Design review of the part built by this model. Coordinates are the model's own, in mm. A direction names the side the tool comes from. Give positions to 0.01 mm unless a question says otherwise; leave off trailing zeros. Order: outer loops, then holes, each group sorted by start corner. A loop starts at its lowest first (then second) coordinate and runs counter-clockwise, first axis right, second up. Notation, with made-up numbers: (75, -35.75) -> (104, -35.75) arc R18 ccw to (104, -18.75) -> close; hole circle Ø6 at (76.5, 34.5). An arc over 180 degrees is marked (long way). One line per item, written item: value. Start each with the question number.
1) Wall thickness on line 1 along Z through (x, y) = (49, 50.5); line 2 along X through (y, z) = (55.5, 20); line 3 along Z through (x, y) = (65, 57): over which ranges is each line inside the solid? List them lowest first. Write a range as from..to.
2) Tool access review of faces 4 (the face through (28, 66, 20)), 5 (the face through (25, 63, 23)), 6 (the face through (50, 68, 47.5)), 7 (the face through (1.5, 21, 35)): name each direction out of +Z, -Z, +X, -X, +Y, -Y from which nothing blocks a thin tool from reaching the whole face with its end or side.
3) Consider section A-A (x = 47). State the section outline as (y, z) points.
4) For pin 1 (7.5 mm diameter, centred on x = 30.5, z = 64, fed in from -Y); pin 2 (1 mm diameter, centred on y = 12.5, z = 35, fed in from -X); pin 3 (2 mm diameter, centred on x = 40, z = 58.5, fed in from -Y), all flat-tipped, find the tip position at first contact; note any pin that passes through.
5) Consider section B-B (z = 48.5). State the section outline as (x, y) points.
6) Consider section C-C (z = 11). State the section outline as (x, y) points.
7) The part is to be moulded in two halves that separate along Y. For faces 1 (the face through (68, 50.3, 51)), 2 (the face through (34.8, 5.7, 1.5)), 3 (the face through (1, 20, 35)), say which applies: released by +Y, released by -Y, zero draft, split by the parting line, or undercut.
from build123d import *

# Parameters (mm, degrees)
BOX079_W               = 5
BOX079_H               = 29
BOX079_DEPTH           = 34
BOX078_W               = 5
BOX078_H               = 28
BOX078_DEPTH           = 32
BOX077_W               = 8
BOX077_H               = 8.3
BOX077_DEPTH           = 6.3
BOX075_W               = 11
BOX075_H               = 10
BOX075_DEPTH           = 11
BOX066_W               = 3
BOX066_H               = 3.5
BOX066_DEPTH           = 12
BOX065_W               = 3
BOX065_H               = 7.5
BOX065_DEPTH           = 17.78
BOX064_W               = 10
BOX064_H               = 8.5
BOX064_DEPTH           = 7.7
CYLINDER036_R          = 1.75
CYLINDER036_DEPTH      = 15
CYLINDER035_R          = 1.75
CYLINDER035_DEPTH      = 15
BOX035_W               = 8
BOX035_H               = 3
BOX035_DEPTH           = 6
BOX034_W               = 8
BOX034_H               = 3
BOX034_DEPTH           = 6
CYLINDER016_R          = 1.7
CYLINDER016_DEPTH      = 15
CYLINDER016_ROLL_ANGLE = 90
CYLINDER015_R          = 1.7
CYLINDER015_DEPTH      = 15
CYLINDER015_ROLL_ANGLE = 90
BOX031_W               = 39
BOX031_H               = 40
BOX031_DEPTH           = 2
BOX032_W               = 34
BOX032_H               = 40
BOX032_DEPTH           = 7
BOX032_PITCH_ANGLE     = 90
BOX033_W               = 34
BOX033_H               = 40
BOX033_DEPTH           = 4
BOX033_PITCH_ANGLE     = 90
BOX028_W               = 15.5
BOX028_H               = 2
BOX028_DEPTH           = 2.5
BOX027_W               = 15.5
BOX027_H               = 2
BOX027_DEPTH           = 2.5
BOX026_W               = 2
BOX026_H               = 2.5
BOX026_DEPTH           = 14
BOX026_ROLL_ANGLE      = 90
BOX025_W               = 2
BOX025_H               = 2.5
BOX025_DEPTH           = 14
BOX025_ROLL_ANGLE      = 90
BOX024_W               = 2.5
BOX024_H               = 2
BOX024_DEPTH           = 51
BOX024_PITCH_ANGLE     = 90
BOX023_W               = 2.5
BOX023_H               = 2
BOX023_DEPTH           = 51
BOX023_PITCH_ANGLE     = 90
BOX022_W               = 2.5
BOX022_H               = 2
BOX022_DEPTH           = 62
BOX021_W               = 2.5
BOX021_H               = 2
BOX021_DEPTH           = 67
BOX020_W               = 62
BOX020_H               = 62
BOX020_DEPTH           = 62
BOX020_ROLL_ANGLE      = 90
PAD005_DEPTH           = 70
SKETCH010_R            = 8.5
POCKET002004_DEPTH     = 5
SKETCH011_W            = 45
SKETCH011_H            = 32
POCKET002005_DEPTH     = 4
FILLET_R               = 3
CHAMFER007_SIZE        = 1.5


with BuildPart() as cube078:
    # Box079 → Box079 (new body)
    with BuildSketch(Plane(origin=(22, 26, 4.1), x_dir=(1, 0, 0), z_dir=(0, 0, 1))):
        with Locations((2.5, 14.5)):
            Rectangle(BOX079_W, BOX079_H)
    extrude(amount=BOX079_DEPTH)


with BuildPart() as cube077:
    # Box078 → Box078 (new body)
    with BuildSketch(Plane(origin=(59, 26, 4.1), x_dir=(1, 0, 0), z_dir=(0, 0, 1))):
        with Locations((2.5, 14)):
            Rectangle(BOX078_W, BOX078_H)
    extrude(amount=BOX078_DEPTH)


with BuildPart() as cube076:
    # Box077 → Box077 (new body)
    with BuildSketch(Plane(origin=(64, 42, 47.5), x_dir=(1, 0, 0), z_dir=(0, 0, 1))):
        with Locations((4, 4.15)):
            Rectangle(BOX077_W, BOX077_H)
    extrude(amount=BOX077_DEPTH)


with BuildPart() as cube074:
    # Box075 → Box075 (new body)
    with BuildSketch(Plane(origin=(44.5, 62, 47.5), x_dir=(1, 0, 0), z_dir=(0, 0, 1))):
        with Locations((5.5, 5)):
            Rectangle(BOX075_W, BOX075_H)
    extrude(amount=BOX075_DEPTH)


with BuildPart() as cube065:
    # Box066 → Box066 (new body)
    with BuildSketch(Plane(origin=(66, 13.5, 44.5), x_dir=(1, 0, 0), z_dir=(0, 0, 1))):
        with Locations((1.5, 1.75)):
            Rectangle(BOX066_W, BOX066_H)
    extrude(amount=BOX066_DEPTH)


with BuildPart() as cube064:
    # Box065 → Box065 (new body)
    with BuildSketch(Plane(origin=(66, 6, 41.5), x_dir=(1, 0, 0), z_dir=(0, 0, 1))):
        with Locations((1.5, 3.75)):
            Rectangle(BOX065_W, BOX065_H)
    extrude(amount=BOX065_DEPTH)


with BuildPart() as cube063:
    # Box064 → Box064 (new body)
    with BuildSketch(Plane(origin=(60, 4, 46.5), x_dir=(1, 0, 0), z_dir=(0, 0, 1))):
        with Locations((5, 4.25)):
            Rectangle(BOX064_W, BOX064_H)
    extrude(amount=BOX064_DEPTH)


with BuildPart() as cylinder068:
    # Cylinder036 → Cylinder036 (new body)
    with BuildSketch(Plane(origin=(24.5, 13.5, -4), x_dir=(1, 0, 0), z_dir=(0, 0, 1))):
        Circle(CYLINDER036_R)
    extrude(amount=CYLINDER036_DEPTH)


with BuildPart() as cylinder067:
    # Cylinder035 → Cylinder035 (new body)
    with BuildSketch(Plane(origin=(35.5, 13.5, 59), x_dir=(1, 0, 0), z_dir=(0, 0, 1))):
        Circle(CYLINDER035_R)
    extrude(amount=CYLINDER035_DEPTH)


with BuildPart() as cube035:
    # Box035 → Box035 (new body)
    with BuildSketch(Plane(origin=(22, 61, 17), x_dir=(1, 0, 0), z_dir=(0, 0, 1))):
        with Locations((4, 1.5)):
            Rectangle(BOX035_W, BOX035_H)
    extrude(amount=BOX035_DEPTH)


with BuildPart() as cube034:
    # Box034 → Box034 (new body)
    with BuildSketch(Plane(origin=(60, 61, 17), x_dir=(1, 0, 0), z_dir=(0, 0, 1))):
        with Locations((4, 1.5)):
            Rectangle(BOX034_W, BOX034_H)
    extrude(amount=BOX034_DEPTH)


with BuildPart() as cylinder051:
    # Cylinder016 → Cylinder016 (new body)
    with BuildSketch(Plane.XY):
        Circle(CYLINDER016_R)
    extrude(amount=CYLINDER016_DEPTH)


with BuildPart() as cylinder051_1:
    # Cylinder016 roll: moved
    add(cylinder051.part.rotate(Axis((0, 0, 0), (1, 0, 0)), CYLINDER016_ROLL_ANGLE))


with BuildPart() as cylinder051_2:
    # Cylinder016 placement: moved
    add(cylinder051_1.part.moved(Location((26, 67, 20))))


with BuildPart() as cylinder050:
    # Cylinder015 → Cylinder015 (new body)
    with BuildSketch(Plane.XY):
        Circle(CYLINDER015_R)
    extrude(amount=CYLINDER015_DEPTH)


with BuildPart() as cylinder050_1:
    # Cylinder015 roll: moved
    add(cylinder050.part.rotate(Axis((0, 0, 0), (1, 0, 0)), CYLINDER015_ROLL_ANGLE))


with BuildPart() as cylinder050_2:
    # Cylinder015 placement: moved
    add(cylinder050_1.part.moved(Location((65, 67, 20))))


with BuildPart() as cube031:
    # Box031 → Box031 (new body)
    with BuildSketch(Plane(origin=(25, 26, 36), x_dir=(1, 0, 0), z_dir=(0, 0, 1))):
        with Locations((19.5, 20)):
            Rectangle(BOX031_W, BOX031_H)
    extrude(amount=BOX031_DEPTH)


with BuildPart() as cube032:
    # Box032 → Box032 (new body)
    with BuildSketch(Plane.XY):
        with Locations((17, 20)):
            Rectangle(BOX032_W, BOX032_H)
    extrude(amount=BOX032_DEPTH)


with BuildPart() as cube032_1:
    # Box032 pitch: moved
    add(cube032.part.rotate(Axis((0, 0, 0), (0, 1, 0)), BOX032_PITCH_ANGLE))


with BuildPart() as cube032_2:
    # Box032 placement: moved
    add(cube032_1.part.moved(Location((22, 26, 38))))


with BuildPart() as cube033:
    # Box033 → Box033 (new body)
    with BuildSketch(Plane.XY):
        with Locations((17, 20)):
            Rectangle(BOX033_W, BOX033_H)
    extrude(amount=BOX033_DEPTH)


with BuildPart() as cube033_1:
    # Box033 pitch: moved
    add(cube033.part.rotate(Axis((0, 0, 0), (0, 1, 0)), BOX033_PITCH_ANGLE))


with BuildPart() as cube033_2:
    # Box033 placement: moved
    add(cube033_1.part.moved(Location((62, 26, 38))))


with BuildPart() as cube028:
    # Box028 → Box028 (new body)
    with BuildSketch(Plane(origin=(1.5, 20, 66), x_dir=(1, 0, 0), z_dir=(0, 0, 1))):
        with Locations((7.75, 1)):
            Rectangle(BOX028_W, BOX028_H)
    extrude(amount=BOX028_DEPTH)


with BuildPart() as cube027:
    # Box027 → Box027 (new body)
    with BuildSketch(Plane(origin=(1.5, 20, 1.5), x_dir=(1, 0, 0), z_dir=(0, 0, 1))):
        with Locations((7.75, 1)):
            Rectangle(BOX027_W, BOX027_H)
    extrude(amount=BOX027_DEPTH)


with BuildPart() as cube026:
    # Box026 → Box026 (new body)
    with BuildSketch(Plane.XY):
        with Locations((1, 1.25)):
            Rectangle(BOX026_W, BOX026_H)
    extrude(amount=BOX026_DEPTH)


with BuildPart() as cube026_1:
    # Box026 roll: moved
    add(cube026.part.rotate(Axis((0, 0, 0), (1, 0, 0)), BOX026_ROLL_ANGLE))


with BuildPart() as cube026_2:
    # Box026 placement: moved
    add(cube026_1.part.moved(Location((15, 20, 1.5))))


with BuildPart() as cube025:
    # Box025 → Box025 (new body)
    with BuildSketch(Plane.XY):
        with Locations((1, 1.25)):
            Rectangle(BOX025_W, BOX025_H)
    extrude(amount=BOX025_DEPTH)


with BuildPart() as cube025_1:
    # Box025 roll: moved
    add(cube025.part.rotate(Axis((0, 0, 0), (1, 0, 0)), BOX025_ROLL_ANGLE))


with BuildPart() as cube025_2:
    # Box025 placement: moved
    add(cube025_1.part.moved(Location((15, 20, 66))))


with BuildPart() as cube024:
    # Box024 → Box024 (new body)
    with BuildSketch(Plane.XY):
        with Locations((1.25, 1)):
            Rectangle(BOX024_W, BOX024_H)
    extrude(amount=BOX024_DEPTH)


with BuildPart() as cube024_1:
    # Box024 pitch: moved
    add(cube024.part.rotate(Axis((0, 0, 0), (0, 1, 0)), BOX024_PITCH_ANGLE))


with BuildPart() as cube024_2:
    # Box024 placement: moved
    add(cube024_1.part.moved(Location((15, 4, 68.5))))


with BuildPart() as cube023:
    # Box023 → Box023 (new body)
    with BuildSketch(Plane.XY):
        with Locations((1.25, 1)):
            Rectangle(BOX023_W, BOX023_H)
    extrude(amount=BOX023_DEPTH)


with BuildPart() as cube023_1:
    # Box023 pitch: moved
    add(cube023.part.rotate(Axis((0, 0, 0), (0, 1, 0)), BOX023_PITCH_ANGLE))


with BuildPart() as cube023_2:
    # Box023 placement: moved
    add(cube023_1.part.moved(Location((15, 4, 4))))


with BuildPart() as cube022:
    # Box022 → Box022 (new body)
    with BuildSketch(Plane(origin=(1.5, 20, 4), x_dir=(1, 0, 0), z_dir=(0, 0, 1))):
        with Locations((1.25, 1)):
            Rectangle(BOX022_W, BOX022_H)
    extrude(amount=BOX022_DEPTH)


with BuildPart() as cube021:
    # Box021 → Box021 (new body)
    with BuildSketch(Plane(origin=(66, 4, 1.5), x_dir=(1, 0, 0), z_dir=(0, 0, 1))):
        with Locations((1.25, 1)):
            Rectangle(BOX021_W, BOX021_H)
    extrude(amount=BOX021_DEPTH)


with BuildPart() as cube020:
    # Box020 → Box020 (new body)
    with BuildSketch(Plane.XY):
        with Locations((31, 31)):
            Rectangle(BOX020_W, BOX020_H)
    extrude(amount=BOX020_DEPTH)


with BuildPart() as cube020_1:
    # Box020 roll: moved
    add(cube020.part.rotate(Axis((0, 0, 0), (1, 0, 0)), BOX020_ROLL_ANGLE))


with BuildPart() as cube020_2:
    # Box020 placement: moved
    add(cube020_1.part.moved(Location((4, 66, 4))))


with BuildPart() as cut094:
    # Sketch009 → Pad005 (new body)
    with BuildSketch(Plane.XY):
        Polygon((0, 20), (15, 20), (15, 4), (70, 4), (70, 70), (0, 70), align=None)
    extrude(amount=PAD005_DEPTH)

    # Cut024: cut Cube020
    add(cube020_2.part, mode=Mode.SUBTRACT)

    # Cut025: cut Cube021
    add(cube021.part, mode=Mode.SUBTRACT)

    # Cut026: cut Cube022
    add(cube022.part, mode=Mode.SUBTRACT)

    # Cut027: cut Cube023
    add(cube023_2.part, mode=Mode.SUBTRACT)

    # Cut028: cut Cube024
    add(cube024_2.part, mode=Mode.SUBTRACT)

    # Cut029: cut Cube025
    add(cube025_2.part, mode=Mode.SUBTRACT)

    # Cut030: cut Cube026
    add(cube026_2.part, mode=Mode.SUBTRACT)

    # Cut031: cut Cube027
    add(cube027.part, mode=Mode.SUBTRACT)

    # Cut032: cut Cube028
    add(cube028.part, mode=Mode.SUBTRACT)

    # Sketch010 → Pocket002004 (cut)
    with BuildSketch(Plane(origin=(0, 0, 0), x_dir=(0, -1, 0), z_dir=(-1, 0, 0))):
        with Locations((-50, 21.5)):
            Circle(SKETCH010_R)
        with Locations((-50, 48.5)):
            Circle(SKETCH010_R)
    extrude(amount=-POCKET002004_DEPTH, mode=Mode.SUBTRACT)

    # Sketch011 → Pocket002005 (cut)
    with BuildSketch(Plane(origin=(0, 70, 0), x_dir=(-1, 0, 0), z_dir=(0, 1, 0))):
        with Locations((-45.5, 20)):
            Rectangle(SKETCH011_W, SKETCH011_H)
    extrude(amount=-POCKET002005_DEPTH, mode=Mode.SUBTRACT)

    # Fusion007: union Cube031, Cube032, Cube033
    add(cube031.part)
    add(cube032_2.part)
    add(cube033_2.part)

    # Cut033: cut Cylinder050
    add(cylinder050_2.part, mode=Mode.SUBTRACT)

    # Cut034: cut Cylinder051
    add(cylinder051_2.part, mode=Mode.SUBTRACT)

    # Cut035: cut Cube034
    add(cube034.part, mode=Mode.SUBTRACT)

    # Cut036: cut Cube035
    add(cube035.part, mode=Mode.SUBTRACT)

    # Fillet
    fillet_edges = [cut094.edges().sort_by_distance(p)[0] for p in [
        (70, 37, 0),
        (0, 45, 0),
        (70, 37, 70),
        (0, 45, 70),
    ]]
    fillet(fillet_edges, radius=FILLET_R)

    # Cut072: cut Cylinder067
    add(cylinder067.part, mode=Mode.SUBTRACT)

    # Cut073: cut Cylinder068
    add(cylinder068.part, mode=Mode.SUBTRACT)

    # Chamfer007
    chamfer007_edges = [cut094.edges().sort_by_distance(p)[0] for p in [
        (33.75, 13.5, 70),
        (22.75, 13.5, 0),
    ]]
    chamfer(chamfer007_edges, length=CHAMFER007_SIZE)

    # Cut076: cut Cube063
    add(cube063.part, mode=Mode.SUBTRACT)

    # Cut077: cut Cube064
    add(cube064.part, mode=Mode.SUBTRACT)

    # Cut078: cut Cube065
    add(cube065.part, mode=Mode.SUBTRACT)

    # Cut085: cut Cube074
    add(cube074.part, mode=Mode.SUBTRACT)

    # Cut087: cut Cube076
    add(cube076.part, mode=Mode.SUBTRACT)

    # Cut088: cut Cube077
    add(cube077.part, mode=Mode.SUBTRACT)

    # Cut089: cut Cube078
    add(cube078.part, mode=Mode.SUBTRACT)


solid = cut094.part
Checked values:
1. line 1: z = 0..4, 36..38, 66..70
1. line 2: x = 22..24.3, 27.7..29, 62..63.3, 66.7..70
1. line 3: z = 0..18.3, 21.7..38, 66..70
2. face 4: +Y
2. face 5: none
2. face 6: +Y, -Y
2. face 7: -Y
3. outline: (4, 0) -> (70, 0) -> (70, 4) -> (6, 4) -> (6, 1.5) -> (4, 1.5) -> close; (4, 68.5) -> (6, 68.5) -> (6, 66) -> (66, 66) -> (66, 58.5) -> (70, 58.5) -> (70, 70) -> (4, 70) -> close; (26, 36) -> (70, 36) -> (70, 47.5) -> (66, 47.5) -> (66, 38) -> (26, 38) -> close
4. pin 1: stops at y = 6
4. pin 2: stops at x = 66
4. pin 3: stops at y = 66
5. outline: (0, 20) -> (1.5, 20) -> (1.5, 22) -> (4, 22) -> (4, 41.5) -> (0, 41.5) -> close; (0, 58.5) -> (4, 58.5) -> (4, 66) -> (44.5, 66) -> (44.5, 70) -> (0, 70) -> close; (55.5, 66) -> (66, 66) -> (66, 50.3) -> (70, 50.3) -> (70, 70) -> (55.5, 70) -> close; (66, 17) -> (69, 17) -> (69, 12.5) -> (70, 12.5) -> (70, 42) -> (66, 42) -> close
6. outline: (0, 20) -> (1.5, 20) -> (1.5, 22) -> (4, 22) -> (4, 66) -> (22, 66) -> (22, 55) -> (27, 55) -> (27, 26) -> (29, 26) -> (29, 66) -> (23, 66) -> (23, 70) -> (0, 70) -> close; (62, 54) -> (64, 54) -> (64, 26) -> (66, 26) -> (66, 6) -> (68.5, 6) -> (68.5, 4) -> (70, 4) -> (70, 70) -> (68, 70) -> (68, 66) -> (62, 66) -> close
7. face 1: undercut
7. face 2: zero draft
7. face 3: released by -Y
